from build123d import *

# Parameters (mm, degrees)
F0_W     = 25
F0_H     = 20
F0_W_2   = 10
F1_DEPTH = 10
F2_DEPTH = 25
F4_D     = 5.2
F4_DEPTH = 1.2
F4_TIP   = 1.5622376095
F3_W     = 2
F3_H     = 2.5
F5_DEPTH = 36.07


with BuildPart() as f1:
    # F0 (on Top) → F1 (new body)
    with BuildSketch(Plane.XY):
        Rectangle(F0_W, F0_H)
        with Locations((-17.5, 0)):
            Rectangle(F0_W_2, F0_H)
        with Locations((17.5, 0)):
            Rectangle(F0_W_2, F0_H)
    extrude(amount=F1_DEPTH)

    # F0 (on Top) → F2 (join)
    with BuildSketch(Plane.XY):
        with Locations((-17.5, 0)):
            Rectangle(F0_W_2, F0_H)
        with Locations((17.5, 0)):
            Rectangle(F0_W_2, F0_H)
    extrude(amount=F2_DEPTH)

    # F4
    with Locations(Plane(origin=(0, 0, 0), x_dir=(1, 0, 0), z_dir=(0, 0, -1))):
        with Locations((0, 0)):
            Hole(F4_D / 2, depth=F4_DEPTH)
            with Locations((0, 0, -(F4_DEPTH + F4_TIP / 2))):  # 118° drill point
                Cone(0, F4_D / 2, F4_TIP, mode=Mode.SUBTRACT)

    # F3 (on face) → F5 (cut)
    with BuildSketch(Plane(origin=(0, 0, 0), x_dir=(1, 0, 0), z_dir=(0, 0, -1))):
        with Locations((18.5, 1.25)):
            Rectangle(F3_W, F3_H)
        with Locations((18.5, -1.25)):
            Rectangle(F3_W, F3_H)
    extrude(amount=-F5_DEPTH, mode=Mode.SUBTRACT)


solid = f1.part
Model file for the job. Use its own axes, mm. A direction names the side the tool comes from. Coordinates: 2 decimals unless noted, no trailing zeros. Order: outer loops, then holes, each group sorted by start corner. A loop starts at its lowest first (then second) coordinate and runs counter-clockwise, first axis right, second up. Notation, with made-up numbers: (53, -25) -> (91, -25) arc R16 ccw to (91, -17) -> close; hole circle Ø7 at (1, 29). An arc over 180 degrees is marked (long way). Return JSON: item names as keys, results as strings. Group by question number.
Item 1: Pull direction Y, two halves, no side cores. Call faces 1 (the conical face through (-0.45, -0.02, 2.49)), 2 (the cylindrical face through (0.338, -2.578, 0.608)), 3 (the flat face through (12.5, 0, 17)), 4 (the flat face through (0.3, 10, 9.5)): pulls with the +Y half, pulls with the -Y half, needs draft (parallel to the pull), parting line crosses it, or undercut.
Item 2: Flat gauge pins, fed straight in: P1, Ø4.5, axis at x = 0, y = 0, coming from the +Z side; P2, Ø1.5, axis at x = 0.5, y = 1.5, coming from the -Z side. Where does each tip first touch, or does it go through?
Item 3: Saw through at C-C on x = -5. Write the cut outline in (y, z).
Item 4: Saw through at B-B on y = -3.75. Write the cut outline in (x, z).
Item 5: Tool access for faces 5 (the flat face through (-12.5, 0, 17)), 6 (the flat face through (19.5, 0, 12)), 7 (the flat face through (17, 0, 25)): list every direction of +Z, -Z, +X, -X, +Y, -Y with a clear straight run to the whole face (end or side of a thin tool).
Item 6: Saw through at A-A on z = 17.25. Write the cut outline in (x, y).
Item 7: Wall check: line 1 along X through (y, z) = (-0.75, 24.25); line 2 along Y through (x, z) = (0, 0.5); line 3 along X through (y, z) = (-1.5, 2.5). Give the ranges that are in metal, low to high. Write a range as [from, to].
Values found:
{
 "1": {"face 1": "undercut", "face 2": "undercut", "face 3": "needs draft", "face 4": "pulls with the +Y half"},
 "2": {"P1": "stops at z = 10", "P2": "stops at z = 1.36"},
 "3": {"outline": "(-10, 0) -> (10, 0) -> (10, 10) -> (-10, 10) -> close"},
 "4": {"outline": "(-22.5, 0) -> (22.5, 0) -> (22.5, 25) -> (12.5, 25) -> (12.5, 10) -> (-12.5, 10) -> (-12.5, 25) -> (-22.5, 25) -> close"},
 "5": {"face 5": "+Z, +Y, -Y", "face 6": "+Z, -Z", "face 7": "+Z, +X, -X, +Y, -Y"},
 "6": {"outline": "(-22.5, -10) -> (-12.5, -10) -> (-12.5, 10) -> (-22.5, 10) -> close; (12.5, -10) -> (22.5, -10) -> (22.5, 10) -> (12.5, 10) -> close; hole (17.5, -2.5) -> (19.5, -2.5) -> (19.5, 2.5) -> (17.5, 2.5) -> close"},
 "7": {"line 1": "x = [-22.5, -12.5], [12.5, 17.5], [19.5, 22.5]", "line 2": "y = [-10, -2.6], [2.6, 10]", "line 3": "x = [-22.5, 17.5], [19.5, 22.5]"}
}
